Read the model definition and answer for the solid it produces. Units are mm, in the model's axes. Face numbers are marked on the shaded views. A direction names the side the tool comes from. Give positions to 0.01 mm unless a question says otherwise; leave off trailing zeros. Order: outer loops, then holes, each group sorted by start corner. A loop starts at its lowest first (then second) coordinate and runs counter-clockwise, first axis right, second up. Notation, with made-up numbers: (50.5, 56) - (106.5, 56) arc R11 cw to (106.5, 77) - close; hole circle Ø8 at (-14.5, -14.75). An arc over 180 degrees is marked (long way). Return JSON: item names as keys, results as strings.
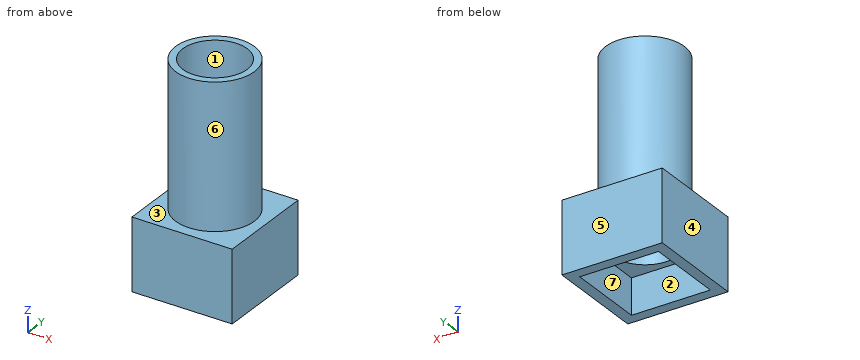
```python
from build123d import *

# Parameters (mm, degrees)
SKETCH_1_W          = 14
SKETCH_1_H          = 14
SKETCH_1_W_2        = 11
SKETCH_1_H_2        = 11
EXTRUDE_1_DEPTH     = 5
SKETCH_2_W          = 14
SKETCH_2_H          = 14
EXTRUDE_2_DEPTH     = 5
SKETCH_3_R          = 5.5
EXTRUDE_3_DEPTH     = 20
SKETCH_4_R          = 4.5
CUT_EXTRUDE_1_DEPTH = 32.591137998


with BuildPart() as part:
    # 草图1 → 凸台-拉伸1 (new body)
    with BuildSketch(Plane.XY):
        Rectangle(SKETCH_1_W, SKETCH_1_H)
        Rectangle(SKETCH_1_W_2, SKETCH_1_H_2, mode=Mode.SUBTRACT)
    extrude(amount=EXTRUDE_1_DEPTH)

    # 草图2 → 凸台-拉伸2 (add)
    with BuildSketch(Plane.XY.offset(5)):
        Rectangle(SKETCH_2_W, SKETCH_2_H)
    extrude(amount=EXTRUDE_2_DEPTH)

    # 草图3 → 凸台-拉伸3 (add)
    with BuildSketch(Plane.XY.offset(10)):
        Circle(SKETCH_3_R)
    extrude(amount=EXTRUDE_3_DEPTH)

    # 草图4 → 切除-拉伸1 (cut, through all)
    with BuildSketch(Plane.XY.offset(30)):
        Circle(SKETCH_4_R)
    extrude(amount=-CUT_EXTRUDE_1_DEPTH, mode=Mode.SUBTRACT)


solid = part.part
```
Q1. For the marked faces 5, 6 and 7, determine the directions among +Z, -Z, +X, -X, +Y, -Y from which every point of the face is accessible in a straight line to the end or side of a thin tool.
Values:
{"face 5": "+Z, -Z, +X, -X, +Y", "face 6": "+Z", "face 7": "-Z"}
Q2. Given pin 1 (3 mm diameter, centred on x = -5.5, z = 17, fed in from -Y); pin 2 (3 mm diameter, centred on y = -4, z = 19, fed in from +X); pin 3 (1.5 mm diameter, centred on x = -1, z = 22, fed in from +Y), each flat-ended and moving along its own axis, determine where each tip first touches the part or whether it passes through.
Values:
{"pin 1": "stops at y = -3.77", "pin 2": "stops at x = 4.9", "pin 3": "stops at y = 5.49"}
Q3. A cutting plane is placed at D-D (x = -5). Write down the section's boundary in (y, z), and give its area (3 significant figures).
Values:
{"outline": "(-7, 0) - (-5.5, 0) - (-5.5, 5) - (5.5, 5) - (5.5, 0) - (7, 0) - (7, 10) - (2.29, 10) - (2.29, 30) - (-2.29, 30) - (-2.29, 10) - (-7, 10) - close", "area": "177 mm²"}
Q4. A cutting plane is placed at A-A (x = 0). Write down the section's boundary in (y, z).
Values:
{"outline": "(-7, 0) - (-5.5, 0) - (-5.5, 5) - (-4.5, 5) - (-4.5, 30) - (-5.5, 30) - (-5.5, 10) - (-7, 10) - close; (4.5, 5) - (5.5, 5) - (5.5, 0) - (7, 0) - (7, 10) - (5.5, 10) - (5.5, 30) - (4.5, 30) - close"}
Q5. A cutting plane is placed at C-C (z = 4.25). Write down the section's boundary in (x, y), and give its area (3 significant figures).
Values:
{"outline": "(-7, -7) - (7, -7) - (7, 7) - (-7, 7) - close; hole (-5.5, -5.5) - (5.5, -5.5) - (5.5, 5.5) - (-5.5, 5.5) - close", "area": "75.0 mm²"}
Q6. Consider L1, parallel to Y at x = 0, z = 21.75; L2, parallel to X at y = 5.25, z = 3.5. Determine where each line is inside the solid, lowest interval first.
Values:
{"L1": "y = -5.5 to -4.5, 4.5 to 5.5", "L2": "x = -7 to -5.5, 5.5 to 7"}
Q7. Determine the mould class of the marked faces 1, 2, 3 and 4 for opening direction X: released by +X, released by -X, zero draft, split by the parting line, or undercut.
Values:
{"face 1": "undercut", "face 2": "undercut", "face 3": "zero draft", "face 4": "released by -X"}
